```python
from build123d import *

# Parameters (mm, degrees)
SKETCH1_W               = 46.355
SKETCH1_H               = 46.355
BOSS_EXTRUDE1_DEPTH     = 127
SKETCH2_R               = 1.397
CUT_EXTRUDE1_DEPTH      = 128
SKETCH4_R               = 3.4925
CUT_EXTRUDE3_DEPTH      = 128
MIRROR2_COPY_1_SKETCH_R = 3.4925
MIRROR2_COPY_1_DEPTH    = 128


with BuildPart() as part:
    # Sketch1 → Boss-Extrude1 (new body)
    with BuildSketch(Plane.XY):
        Rectangle(SKETCH1_W, SKETCH1_H)
    extrude(amount=BOSS_EXTRUDE1_DEPTH)

    # Sketch2 → Cut-Extrude1 (cut, through all)
    with BuildSketch(Plane.XY.offset(127)):
        Circle(SKETCH2_R)
    extrude(amount=-CUT_EXTRUDE1_DEPTH, mode=Mode.SUBTRACT)

    # Sketch4 → Cut-Extrude3 (cut, through all)
    with BuildSketch(Plane.XY.offset(127)):
        with Locations((14.601896453, 14.601896453)):
            Circle(SKETCH4_R)
    cut_extrude3 = extrude(amount=-CUT_EXTRUDE3_DEPTH, mode=Mode.SUBTRACT)

    # Mirror1: Cut-Extrude3 across plane
    add(cut_extrude3.mirror(Plane.ZX), mode=Mode.SUBTRACT)

    # Mirror2: Cut-Extrude3 across plane
    add(cut_extrude3.mirror(Plane(origin=(0, 0, 0), x_dir=(0, 0, 1), z_dir=(1, 0, 0))), mode=Mode.SUBTRACT)

    # Mirror2 copy 1 sketch → Mirror2 copy 1 (cut, through all)
    with BuildSketch(Plane(origin=(0, 0, 127), x_dir=(-1, 0, 0), z_dir=(0, 0, 1))):
        with Locations((14.601896453, 14.601896453)):
            Circle(MIRROR2_COPY_1_SKETCH_R)
    extrude(amount=-MIRROR2_COPY_1_DEPTH, mode=Mode.SUBTRACT)

    # Sketch5 → Cut-Revolve1 (revolve, cut)
    with BuildSketch(Plane(origin=(0, 0, 0), x_dir=(0, 0, -1), z_dir=(1, 0, 0))):
        Polygon((0, 14.601896453), (-44.712215564, 14.601896453), (-70.584924633, 2.078286108), (-70.584924633, 13.343436946), (-87.296961591, 13.343436946), (-127, 2.078286108), (-127, 0), (0, 0), align=None)
    revolve(axis=Axis((0, 0, 127), (0, 0, -1)), mode=Mode.SUBTRACT)


solid = part.part
```
Source: CAD feature listing. Evaluate the final solid. Frame: model axes, mm. A direction names the side the tool comes from. Coordinates: 2 decimals unless noted, no trailing zeros. Loops run counter-clockwise (first coordinate to the right, second up) from the corner with the lowest first, then second, coordinate; pieces in that order, holes last. Notation, with made-up numbers: (-0.5, 2.25) - (58.5, 2.25) arc R6 ccw to (58.5, 12.25) - close; hole circle Ø4 at (-26.5, 65). An arc over 180 degrees is marked (long way). Answer as CSV lines item,"result".
1. Section B-B (x = 0). Return loops of the section in (y, z), then the cut area to 3 significant figures.
Established:
outline,"(-23.18, 0) - (-14.6, 0) - (-14.6, 44.71) - (-2.08, 70.58) - (-13.34, 70.58) - (-13.34, 87.3) - (-2.08, 127) - (-23.18, 127) - close; (2.08, 70.58) - (14.6, 44.71) - (14.6, 0) - (23.18, 0) - (23.18, 127) - (2.08, 127) - (13.34, 87.3) - (13.34, 70.58) - close"
area,"3,090 mm2"
2. Ray query, line 1 (X direction, y = 12.5, z = 22); line 2 (X direction, y = 17.5, z = 59); line 3 (Y direction, x = 15.5, z = 91.5). Return the intervals inside material, ascending.
Established:
line 1,"x = -23.18 to -17.39, -11.81 to -7.55, 7.55 to 11.81, 17.39 to 23.18"
line 2,"x = -23.18 to -16.55, -12.65 to 12.65, 16.55 to 23.18"
line 3,"y = -23.18 to -17.98, -11.23 to 11.23, 17.98 to 23.18"
3. Section A-A (z = 36). Return loops of the section in (x, y) (1 decimal), then the cut area to 3 significant figures.
Established:
outline,"(-23.2, -23.2) - (23.2, -23.2) - (23.2, 23.2) - (-23.2, 23.2) - close; hole circle Ø7 at (-14.6, -14.6); hole circle Ø7 at (-14.6, 14.6); hole circle Ø29.2 at (0, 0); hole circle Ø7 at (14.6, -14.6); hole circle Ø7 at (14.6, 14.6)"
area,"1,330 mm2"
4. Mould query, pull axis Y, two halves, no side actions, for faces 3 (the cylindrical face through (4.386, 13.928, 22.669)), 4 (the flat face through (0, -23.178, 63)), 5 (the flat face through (-23.178, 0, 63)). Classes: released by +Y, released by -Y, zero draft, split by the parting line, or undercut.
Established:
face 3,"undercut"
face 4,"released by -Y"
face 5,"zero draft"
5. Reachability of faces 1 (the conical face through (0.302, -6.854, 60.704)), 2 (the cylindrical face through (-13, -3, 79)) from +Z, -Z, +X, -X, +Y, -Y: full face, straight path, thin tool, end or side. Return the list, or none.
Established:
face 1,"-Z"
face 2,"none"
6. Contact query for flat-ended pins moving along their axis: pin 1 (24 mm diameter, centred on x = 0, y = 0, fed in from -Z); pin 2 (4 mm diameter, centred on x = -14.6, y = 14.6, fed in from +Z); pin 3 (12 mm diameter, centred on x = -4.5, y = 1.5, fed in from -Z); pin 4 (17.5 mm diameter, centred on x = 0, y = 0, fed in from -Z). Output: stop coordinate, or through.
Established:
pin 1,"stops at z = 50.09"
pin 2,"passes through"
pin 3,"stops at z = 52.68"
pin 4,"stops at z = 56.8"
7. Section D-D (z = 56). Return loops of the section in (x, y) (1 decimal).
Established:
outline,"(-23.2, -23.2) - (23.2, -23.2) - (23.2, 23.2) - (-23.2, 23.2) - close; hole circle Ø7 at (-14.6, -14.6); hole circle Ø7 at (-14.6, 14.6); hole circle Ø18.3 at (0, 0); hole circle Ø7 at (14.6, -14.6); hole circle Ø7 at (14.6, 14.6)"
